Geometry: final body of the model. Coordinates: model frame, mm. A direction names the side the tool comes from. Give positions to 0.01 mm unless a question says otherwise; leave off trailing zeros. Order: outer loops, then holes, each group sorted by start corner. A loop starts at its lowest first (then second) coordinate and runs counter-clockwise, first axis right, second up. Notation, with made-up numbers: M 78,46.25 L 108,46.25 A22 ccw 108,65.25 Z; hole C 32.25,72 d7. An arc over 180 degrees is marked long. Use CSV: the item, a comma, the result in double quotes.
```python
from build123d import *

# Parameters (mm, degrees)
SKETCH1_W           = 41
SKETCH1_H           = 70
SKETCH1_R           = 3.3
BOSS_EXTRUDE1_DEPTH = 8
SKETCH2_R           = 5.5
CUT_EXTRUDE1_DEPTH  = 4.2
CHAMFER2_SIZE       = 3.2
FILLET1_R           = 4
CHAMFER4_SIZE       = 0.5
SKETCH4_R           = 5.1
CUT_EXTRUDE3_DEPTH  = 9
SKETCH5_R           = 10
CUT_EXTRUDE4_DEPTH  = 4.2


with BuildPart() as part:
    # Sketch1 → Boss-Extrude1 (new body)
    with BuildSketch(Plane(origin=(0, 0, 0), x_dir=(1, 0, 0), z_dir=(0, 1, 0))):
        Rectangle(SKETCH1_W, SKETCH1_H)
        with Locations((0, 17.5)):
            Circle(SKETCH1_R, mode=Mode.SUBTRACT)
        with Locations((0, -17.5)):
            Circle(SKETCH1_R, mode=Mode.SUBTRACT)
    extrude(amount=BOSS_EXTRUDE1_DEPTH)

    # Sketch2 → Cut-Extrude1 (cut)
    with BuildSketch(Plane(origin=(0, 8, 0), x_dir=(1, 0, 0), z_dir=(0, 1, 0))):
        with Locations((0, -17.5)):
            Circle(SKETCH2_R)
    extrude(amount=-CUT_EXTRUDE1_DEPTH, mode=Mode.SUBTRACT)

    # Chamfer2
    chamfer2_edges = [part.edges().sort_by_distance(p)[0] for p in [
        (-3.3, 8, -17.5),
    ]]
    chamfer(chamfer2_edges, length=CHAMFER2_SIZE)

    # Fillet1
    fillet1_edges = [part.edges().sort_by_distance(p)[0] for p in [
        (20.5, 4, 35),
        (-20.5, 4, 35),
        (-20.5, 4, -35),
        (20.5, 4, -35),
    ]]
    fillet(fillet1_edges, radius=FILLET1_R)

    # Chamfer4
    chamfer4_edges = [part.edges().sort_by_distance(p)[0] for p in [
        (0, 0, 35),
        (0, 8, 35),
        (20.5, 0, 0),
        (-20.5, 0, 0),
        (0, 0, -35),
        (-19.328427125, 0, -33.828427125),
        (19.328427125, 0, -33.828427125),
        (19.328427125, 0, 33.828427125),
        (-19.328427125, 0, 33.828427125),
        (-20.5, 8, 0),
        (20.5, 8, 0),
        (0, 8, -35),
        (-19.328427125, 8, -33.828427125),
        (19.328427125, 8, -33.828427125),
        (19.328427125, 8, 33.828427125),
        (-19.328427125, 8, 33.828427125),
    ]]
    chamfer(chamfer4_edges, length=CHAMFER4_SIZE)

    # Sketch4 → Cut-Extrude3 (cut, through all)
    with BuildSketch(Plane(origin=(0, 8, 0), x_dir=(1, 0, 0), z_dir=(0, 1, 0))):
        Circle(SKETCH4_R)
    extrude(amount=-CUT_EXTRUDE3_DEPTH, mode=Mode.SUBTRACT)

    # Sketch5 → Cut-Extrude4 (cut)
    with BuildSketch(Plane(origin=(0, 8, 0), x_dir=(1, 0, 0), z_dir=(0, 1, 0))):
        Circle(SKETCH5_R)
    extrude(amount=-CUT_EXTRUDE4_DEPTH, mode=Mode.SUBTRACT)


solid = part.part
```
1. Section B-B, the plane z = -17.5. Return the cut outline in (x, y), plus the area to 3 significant figures.
Answer:
outline,"M -20.5,0.5 L -20,0 L -3.3,0 L -3.3,4.8 L -6.5,8 L -20,8 L -20.5,7.5 Z; M 3.3,0 L 20,0 L 20.5,0.5 L 20.5,7.5 L 20,8 L 6.5,8 L 3.3,4.8 Z"
area,"264 mm2"
2. Line query: line 1 (Z direction, x = 0, y = 2.9); line 2 (Z direction, x = 0, y = 5.7); line 3 (X direction, y = 1.5, z = 0). Output: solid intervals per line, ascending.
Answer:
line 1,"-35 to -20.8, -14.2 to -5.1, 5.1 to 14.2, 20.8 to 35"
line 2,"-35 to -21.7, -13.3 to -10, 10 to 12, 23 to 35"
line 3,"-20.5 to -5.1, 5.1 to 20.5"
3. Section C-C, the plane y = 3. Return the cut outline in (x, z).
Answer:
outline,"M -20.5,-31 A4 ccw -16.5,-35 L 16.5,-35 A4 ccw 20.5,-31 L 20.5,31 A4 ccw 16.5,35 L -16.5,35 A4 ccw -20.5,31 Z; hole C 0,0 d10.2; hole C 0,-17.5 d6.6; hole C 0,17.5 d6.6"
4. Section D-D, the plane z = 8. Return the cut outline in (x, y).
Answer:
outline,"M -20.5,0.5 L -20,0 L 20,0 L 20.5,0.5 L 20.5,7.5 L 20,8 L 6,8 L 6,3.8 L -6,3.8 L -6,8 L -20,8 L -20.5,7.5 Z"
5. Reachability of faces 5 (the face through (19.297, 4.049, 33.859)), 6 (the face through (-2, 3.8, -5)) from +Z, -Z, +X, -X, +Y, -Y: full face, straight path, thin tool, end or side. Return the list, or none.
Answer:
face 5,"+Z, +X, +Y, -Y"
face 6,"+Y"
6. Section A-A, the plane x = 0. Give the number of separate pieces and of enclosed holes in the cut face, plus the area to 3 significant figures.
Answer:
separate pieces,"4"
enclosed holes,"0"
area,"302 mm2"
7. Pull-direction query (Z, two-part tool) for faces 1 (the face through (-19.05, 7.86, -33.6)), 2 (the face through (-19.099, 0.135, 33.542)), 3 (the face through (0, 3.8, 21)), 4 (the face through (-2.17, 5.93, 9.76)); classes: +Z half, -Z half, draft (parallel to the pull), parting line (faces both ways), or undercut.
Answer:
face 1,"-Z half"
face 2,"+Z half"
face 3,"undercut"
face 4,"undercut"
8. Pin query (flat end, axial travel): pin 1 Ø4 at (x, z) = (0, -17.5) entering from +Y; pin 2 Ø3.5 at (x, z) = (-2.5, 15.5) entering from +Y. Return the tip coordinate at first contact, or that it passes through.
Answer:
pin 1,"through"
pin 2,"y = 3.8"
